Build history of the part. All positions in model axes, mm. Face numbers are marked on the shaded views. A direction names the side the tool comes from. Give positions to 0.01 mm unless a question says otherwise; leave off trailing zeros. Write each loop counter-clockwise with the first axis right and the second up, starting at its lowest first coordinate (ties: lowest second). Pieces come first, ordered by that corner, then holes. Notation, with made-up numbers: (-4, -22) -> (45, -22) arc R28 cw to (45, 13) -> close; hole circle Ø10 at (89, 68.25). An arc over 180 degrees is marked (long way). Put each result on its own line as item: value.
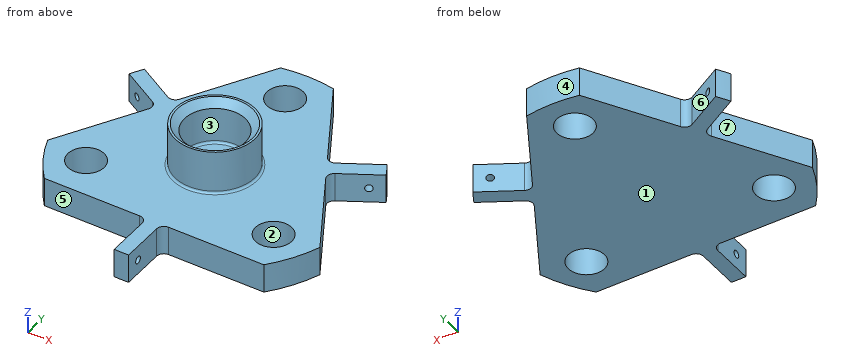
from build123d import *

# Parameters (mm, degrees)
SKETCH1_R           = 27.5
SKETCH1_R_2         = 21
BOSS_EXTRUDE1_DEPTH = 50
SKETCH1_3_R         = 100
SKETCH1_3_R_2       = 27.5
SKETCH1_3_R_3       = 21
BOSS_EXTRUDE2_DEPTH = 20
CHAMFER1_SIZE       = 5
FILLET1_R           = 1.5
SKETCH10_R          = 12.5
CUT_EXTRUDE1_DEPTH  = 20
SKETCH12_W          = 90
SKETCH12_H          = 35
CUT_EXTRUDE3_DEPTH  = 151
SKETCH13_R          = 2.5
CUT_EXTRUDE4_DEPTH  = 151.840188116
SKETCH14_R          = 2.5
CUT_EXTRUDE5_DEPTH  = 150.526515224
SKETCH15_R          = 2.5
CUT_EXTRUDE6_DEPTH  = 151.840188116


with BuildPart() as part:
    # Sketch1 → Boss-Extrude1 (new body)
    with BuildSketch(Plane.XY):
        Circle(SKETCH1_R)
        Circle(SKETCH1_R_2, mode=Mode.SUBTRACT)
    extrude(amount=BOSS_EXTRUDE1_DEPTH)

    # Sketch1<3> → Boss-Extrude2 (add)
    # profile 1 of 2: a face of its own
    with BuildSketch(Plane.XY):
        Circle(SKETCH1_3_R)
        Circle(SKETCH1_3_R_2, mode=Mode.SUBTRACT)
    # profile 2 of 2: a face of its own
    with BuildSketch(Plane.XY):
        Circle(SKETCH1_3_R_3)
    extrude(amount=BOSS_EXTRUDE2_DEPTH)

    # Chamfer1
    chamfer1_edges = [part.edges().sort_by_distance(p)[0] for p in [
        (-21, 0, 50),
    ]]
    chamfer(chamfer1_edges, length=CHAMFER1_SIZE)

    # Fillet1
    fillet1_edges = [part.edges().sort_by_distance(p)[0] for p in [
        (-21, 0, 20),
        (-27.5, 0, 20),
    ]]
    fillet(fillet1_edges, radius=FILLET1_R)

    # Sketch10 → Cut-Extrude1 (cut)
    with BuildSketch(Plane.XY.offset(20)):
        with Locations((0, 75)):
            Circle(SKETCH10_R)
        with Locations((64.951905284, -37.5)):
            Circle(SKETCH10_R)
        with Locations((-64.951905284, -37.5)):
            Circle(SKETCH10_R)
    extrude(amount=-CUT_EXTRUDE1_DEPTH, mode=Mode.SUBTRACT)

    # Sketch12 → Cut-Extrude3 (cut, through all)
    with BuildSketch(Plane(origin=(0, 0, 0), x_dir=(-1, 0, 0), z_dir=(0, 0, -1))):
        with BuildLine():
            Line((-15, -130), (-15, -70))
            ThreePointArc((-15, -70), (-10, -65), (-5, -70))
            Line((-5, -70), (-5, -130))
            ThreePointArc((-5, -130), (-10, -135), (-15, -130))
        make_face()
        Polygon((-61.291651246, 23.839745962), (-91.602540378, 41.339745962), (-136.602540378, -36.602540378), (-106.291651246, -54.102540378), align=None)
        with BuildLine():
            Line((5, -130), (5, -70))
            ThreePointArc((5, -70), (10, -65), (15, -70))
            Line((15, -70), (15, -130))
            ThreePointArc((15, -130), (10, -135), (5, -130))
        make_face()
        with Locations((-55, -82.5)):
            Rectangle(SKETCH12_W, SKETCH12_H)
        with Locations((55, -82.5)):
            Rectangle(SKETCH12_W, SKETCH12_H)
        Polygon((-51.291651246, 41.160254038), (-81.602540378, 58.660254038), (-36.602540378, 136.602540378), (-6.291651246, 119.102540378), align=None)
        with BuildLine():
            Line((-110.083302492, 69.330127019), (-58.121778265, 39.330127019))
            ThreePointArc((-58.121778265, 39.330127019), (-51.291651246, 41.160254038), (-53.121778265, 47.990381057))
            Line((-53.121778265, 47.990381057), (-105.083302492, 77.990381057))
            ThreePointArc((-105.083302492, 77.990381057), (-111.913429511, 76.160254038), (-110.083302492, 69.330127019))
        make_face()
        with BuildLine():
            Line((-120.083302492, 52.009618943), (-68.121778265, 22.009618943))
            ThreePointArc((-68.121778265, 22.009618943), (-61.291651246, 23.839745962), (-63.121778265, 30.669872981))
            Line((-63.121778265, 30.669872981), (-115.083302492, 60.669872981))
            ThreePointArc((-115.083302492, 60.669872981), (-121.913429511, 58.839745962), (-120.083302492, 52.009618943))
        make_face()
        Polygon((51.291651246, 41.160254038), (81.602540378, 58.660254038), (36.602540378, 136.602540378), (6.291651246, 119.102540378), align=None)
        Polygon((61.291651246, 23.839745962), (91.602540378, 41.339745962), (136.602540378, -36.602540378), (106.291651246, -54.102540378), align=None)
        with BuildLine():
            Line((115.083302492, 60.669872981), (63.121778265, 30.669872981))
            ThreePointArc((63.121778265, 30.669872981), (61.291651246, 23.839745962), (68.121778265, 22.009618943))
            Line((68.121778265, 22.009618943), (120.083302492, 52.009618943))
            ThreePointArc((120.083302492, 52.009618943), (121.913429511, 58.839745962), (115.083302492, 60.669872981))
        make_face()
        with BuildLine():
            Line((105.083302492, 77.990381057), (53.121778265, 47.990381057))
            ThreePointArc((53.121778265, 47.990381057), (51.291651246, 41.160254038), (58.121778265, 39.330127019))
            Line((58.121778265, 39.330127019), (110.083302492, 69.330127019))
            ThreePointArc((110.083302492, 69.330127019), (111.913429511, 76.160254038), (105.083302492, 77.990381057))
        make_face()
    extrude(amount=-CUT_EXTRUDE3_DEPTH, mode=Mode.SUBTRACT)

    # Sketch13 → Cut-Extrude4 (cut, through all)
    with BuildSketch(Plane(origin=(2.5, -4.330127019, 0), x_dir=(0.8660254037844378, 0.5000000000000017, 0), z_dir=(0.5000000000000016, -0.8660254037844377, 0))):
        with Locations((89.874921777, 10)):
            Circle(SKETCH13_R)
    extrude(amount=-CUT_EXTRUDE4_DEPTH, mode=Mode.SUBTRACT)

    # Sketch14 → Cut-Extrude5 (cut, through all)
    with BuildSketch(Plane.ZY.offset(5)):
        with Locations((10, -89.874921777)):
            Circle(SKETCH14_R)
    extrude(amount=-CUT_EXTRUDE5_DEPTH, mode=Mode.SUBTRACT)

    # Sketch15 → Cut-Extrude6 (cut, through all)
    with BuildSketch(Plane(origin=(-2.5, -4.330127019, 0), x_dir=(0.8660254037844392, -0.49999999999999906, 0), z_dir=(-0.49999999999999906, -0.8660254037844392, 0))):
        with Locations((-89.874921777, 10)):
            Circle(SKETCH15_R)
    extrude(amount=-CUT_EXTRUDE6_DEPTH, mode=Mode.SUBTRACT)


solid = part.part
1) Slice it at B-B (y = -37.5). Write the cut outline in (x, z).
Filled sheet:
outline: (-92.7, 0) -> (-77.45, 0) -> (-77.45, 20) -> (-92.7, 20) -> close; (-52.45, 0) -> (52.45, 0) -> (52.45, 20) -> (-52.45, 20) -> close; (77.45, 0) -> (92.7, 0) -> (92.7, 20) -> (77.45, 20) -> close
2) Pull direction Y, two halves, no side cores. Call the marked faces 1, 2, 3 and 4: released by +Y, released by -Y, zero draft, split by the parting line, or undercut.
Filled sheet:
face 1: zero draft
face 2: undercut
face 3: undercut
face 4: released by +Y
3) Slice it at A-A (x = 0). Write the cut outline in (y, z), plus the area to 3 significant figures.
Filled sheet:
outline: (-100, 0) -> (62.5, 0) -> (62.5, 20) -> (29, 20) arc R1.5 cw to (27.5, 21.5) -> (27.5, 50) -> (26, 50) -> (21, 45) -> (21, 21.5) arc R1.5 cw to (19.5, 20) -> (-19.5, 20) arc R1.5 cw to (-21, 21.5) -> (-21, 45) -> (-26, 50) -> (-27.5, 50) -> (-27.5, 21.5) arc R1.5 cw to (-29, 20) -> (-100, 20) -> close; (87.5, 0) -> (100, 0) -> (100, 20) -> (87.5, 20) -> close; hole circle Ø5 at (-89.87, 10)
area: 3,850 mm2
4) Slice it at D-D (z = 34). Write the cut outline in (x, y), plus the area to 3 significant figures.
Filled sheet:
outline: circle Ø55 at (0, 0); hole circle Ø42 at (0, 0)
area: 990 mm2
5) Pin check, flat tips, straight feed: pin 1 (4 mm diameter, centred on x = 24, z = 16, fed in from -Y); pin 2 (12 mm diameter, centred on x = 30, y = 4, fed in from -Z); pin 3 (19.5 mm diameter, centred on x = -5.5, y = 2, fed in from +Z); pin 4 (1.5 mm diameter, centred on x = -9, z = 35.5, fed in from +Y). Stop position of each tip, or through.
Filled sheet:
pin 1: y = -65
pin 2: z = 0
pin 3: z = 20
pin 4: y = 26.23
6) Wall check: L1, parallel to Y at x = 0, z = 10; L2, parallel to X at y = -30.5, z = 18; L3, parallel to Y at x = -1.75, z = 10. Give the ranges that are in metal, low to high.
Filled sheet:
L1: -100 to -92.37, -87.37 to 62.5, 87.5 to 100
L2: -92.66 to -75.31, -54.6 to 54.6, 75.31 to 92.66
L3: -99.98 to -92.37, -87.37 to 62.62, 87.38 to 99.98
7) Tool access for the marked faces 5, 6 and 7: list every direction of +Z, -Z, +X, -X, +Y, -Y with a clear straight run to the whole face (end or side of a thin tool).
Filled sheet:
face 5: +Z, -Z, -X, -Y
face 6: +Z, -Z, +Y
face 7: +Z, -Z, -X
8) Slice it at C-C (x = -55.5). Write the cut outline in (y, z).
Filled sheet:
outline: (-65, 0) -> (-45.68, 0) -> (-45.68, 20) -> (-65, 20) -> close; (-29.32, 0) -> (38.66, 0) -> (38.66, 20) -> (-29.32, 20) -> close
